Autodesk Inventor part; units mm, degrees
ref_plane "YZ Plane" through (0, 0, 0) normal (1, 0, 0) x (0, 1, 0)
ref_plane "XZ Plane" through (0, 0, 0) normal (0, 1, 0) x (-1, 0, 0)
ref_plane "XY Plane" through (0, 0, 0) normal (0, 0, 1) x (1, 0, 0)
sketch "Sketch1" plane through (0, 0, 0) normal (0, 1, 0) x (-1, 0, 0)
  circle A0 centre (0, 0) radius 7.5
  circle A1 centre (0, 0) radius 2.5
  dimension "d0" = 15
  dimension "d1" = 5
extrude "Extrusion1" add sketch "Sketch1" along normal blind 1.5 contours A0 | A1
sketch "Sketch2" plane through (0, 1.5, 0) normal (0, 1, 0) x (1, 0, 0)
  circle A0 centre (0, 0) radius 2.5
  circle A1 centre (0, 0) radius 7.5
  line L0 (-0.9798, 2.3) -> (-7.1386, 2.3)
  circle A2 centre (0, 0) radius 7.5
  line L1 (-2.3, 0.9798) -> (-2.3, 7.1386)
  line L2 (-2.3, 7.1386) -> (-7.1386, 2.3)
  line L3 (-3.8, 2.3) -> (-3.8, 6.4661)
  line L4 (-2.3, -0.9798) -> (-2.3, -7.1386)
  line L5 (-0.9798, -2.3) -> (-7.1386, -2.3)
  line L6 (-2.3, -3.8) -> (-6.4661, -3.8)
  line L7 (-7.1386, -2.3) -> (-2.3, -7.1386)
  line L8 (0.9798, -2.3) -> (7.1386, -2.3)
  line L9 (2.3, -0.9798) -> (2.3, -7.1386)
  line L10 (3.8, -2.3) -> (3.8, -6.4661)
  line L11 (2.3, -7.1386) -> (7.1386, -2.3)
  line L12 (2.3, 0.9798) -> (2.3, 7.1386)
  line L13 (0.9798, 2.3) -> (7.1386, 2.3)
  line L14 (2.3, 3.8) -> (6.4661, 3.8)
  line L15 (7.1386, 2.3) -> (2.3, 7.1386)
  point P0 (2.3, -2.3)
  point P1 (2.3, -7.1386)
  point P2 (2.3, 2.3)
  point P3 (-2.3, 2.3)
  point P4 (-2.3, -2.3)
  dimension "d4" = 5
  dimension "d5" = 2.3
  dimension "d6" = 2.3
  dimension "d7" = 6.8429
  dimension "d8" = 1.5
  dimension "d11" = 360
extrude "Extrusion2" add sketch "Sketch2" along normal blind 4.5 contours L12 L14 L15 L13 | L8 L10 L11 L9 | L15 L14 A1 | L11 L10 A1 | L0 L3 L2 L1 | L4 L6 L7 L5 | L2 L3 A1 | L7 L6 A1 picked at (6.5762, 2.972) picked at (2.972, -6.5762) picked at (-2.972, 6.5762) picked at (-6.5762, -2.972)
sketch "Sketch3" plane through (0, 1.5, 0) normal (0, 1, 0) x (1, 0, 0)
  circle A0 centre (0, 0) radius 2.5
  dimension "d15" = 5
extrude "Extrusion3" add sketch "Sketch3" along normal blind 38.5
sketch "Sketch4" plane through (0, 0, 0) normal (0, -1, 0) x (1, 0, 0)
  point P0 (0, 0)
  point P1 (0, 0)
hole "Hole1" [suppressed]
fillet "Fillet1" [suppressed]
properties part number "claw_nut"
Geometry: final body of the model. Coordinates: model frame, mm. A direction names the side the tool comes from. Give positions to 0.01 mm unless a question says otherwise; leave off trailing zeros. Write each loop counter-clockwise with the first axis right and the second up, starting at its lowest first coordinate (ties: lowest second). Pieces come first, ordered by that corner, then holes.
(1) Cut plane C-C, the plane y = 17.5. Return loops of the section in (x, z).
(2) Cut plane A-A, the plane x = 0. Return loops of the section in (y, z), then the cut area to 3 significant figures.
(3) Ray query, line 1 (Y direction, x = -2.5, z = 3.25); line 2 (Y direction, x = 1.5, z = 3.25); line 3 (Z direction, x = 0, y = 18.5). Return the intervals inside material, ascending.
(4) First-contact query: P1, Ø0.8, axis at x = 3, z = 4.5, coming from the +Y side; P2, Ø4.5, axis at x = 4.5, y = 4, coming from the -Z side; P3, Ø4, axis at y = 12.5, z = -1.5, coming from the -X side. Flat tips, straight axial feed; report the tip coordinate or a pass-through.
(5) Mould query, pull axis X, two halves, no side actions, for faces 1 (the flat face through (3.8, 4, 4)), 2 (the flat face through (0, 40, 0)), 3 (the flat face through (2.3, 4, -3)). Classes: released by +X, released by -X, zero draft, split by the parting line, or undercut.
(6) Cut plane B-B, the plane z = 4.5. Return loops of the section in (x, y).
(7) Access query for faces 4 (the flat face through (-4, 4, 3.8)), 5 (the flat face through (3, 4, 2.3)), 6 (the flat face through (-3.8, 4, -4)). Directions: +Z, -Z, +X, -X, +Y, -Y. A direction counts if a zero-diameter tool reaches every point of the face in a straight line with its end or side. Return the directions, or none.
Values follow:
1. outline: circle Ø5 at (0, 0)
2. outline: (0, -7.5) - (1.5, -7.5) - (1.5, -2.5) - (40, -2.5) - (40, 2.5) - (1.5, 2.5) - (1.5, 7.5) - (0, 7.5) - close
2. area: 215 mm2
3. line 1: y = 0 to 6
3. line 2: y = 0 to 1.5
3. line 3: z = -2.5 to 2.5
4. P1: stops at y = 6
4. P2: stops at z = -3.8
4. P3: stops at x = -2.5
5. face 1: released by +X
5. face 2: zero draft
5. face 3: undercut
6. outline: (-6, 0) - (6, 0) - (6, 1.5) - (3.8, 1.5) - (3.8, 6) - (2.3, 6) - (2.3, 1.5) - (-6, 1.5) - close
7. face 4: +Z, -X, +Y
7. face 5: +X, +Y
7. face 6: -Z, -X, +Y
